Here's how the part is built. I have some questions about the finished solid (model axes, mm). Face numbers are marked on the shaded views. A direction names the side the tool comes from. Coordinates: 2 decimals unless noted, no trailing zeros. Order: outer loops, then holes, each group sorted by start corner. A loop starts at its lowest first (then second) coordinate and runs counter-clockwise, first axis right, second up. Notation, with made-up numbers: (-2, 45.25) - (16, 45.25) arc R24 ccw to (16, 76.25) - close; hole circle Ø1 at (23, -5.75). An arc over 180 degrees is marked (long way). Answer in a Markdown table with one row per item. Add a question column.
Item 1: If I drill on line 1 along X through (y, z) = (172, 53); line 2 along Z through (x, y) = (26.5, 202.5), over which ranges is the centre line in solid material (lowest first)? Write a range as from..to.
Item 2: I want a section at C-C (z = -3). Please give me the cut outline in (x, y), plus the area to 3 significant figures.
Item 3: Will these pins go through, and if not, where does the flat tip stop? pin 1 Ø12 at (x, z) = (34, -24.5) entering from +Y; pin 2 Ø2 at (x, y) = (55.5, 202.5) entering from +Z.
Item 4: I want a section at A-A (y = 42). Please give me the cut outline in (x, z), plus the area to 3 significant figures.
Item 5: I want a section at B-B (x = 53). Please give me the cut outline in (y, z).
Item 6: On a 3-axis mill with a long thin cutter (end or side, diameter ignored), from which of +Z, -Z, +X, -X, +Y, -Y can I reach the whole of each face in a straight line? I mean the marked faces 1 and 2. Say none if no direction works.
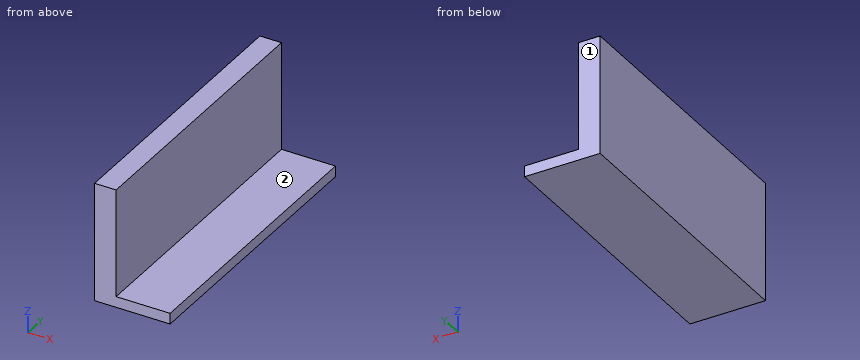
Autodesk Inventor part; units mm, degrees
ref_plane "YZ Plane" through (0, 0, 0) normal (1, 0, 0) x (0, 1, 0)
ref_plane "XZ Plane" through (0, 0, 0) normal (0, 1, 0) x (-1, 0, 0)
ref_plane "XY Plane" through (0, 0, 0) normal (0, 0, 1) x (1, 0, 0)
sketch "Sketch1" plane through (0, 0, 0) normal (0, 1, 0) x (-1, 0, 0)
  line L0 (-3.913, 66.9565) -> (-23.913, 66.9565)
  line L1 (-23.913, 66.9565) -> (-23.913, -43.0435)
  line L2 (-23.913, -43.0435) -> (-3.913, -43.0435)
  line L3 (-3.913, -43.0435) -> (-3.913, 66.9565)
  line L4 (53.6957, 6.9565) -> (-3.913, 6.9565)
  line L5 (-3.913, 6.9565) -> (-3.913, -18.0435)
  line L6 (-3.913, -18.0435) -> (48.6957, -18.0435)
  point P0 (0, 0)
  dimension "d0" = 110
  dimension "d1" = 20
  dimension "d3" = 60
extrude "Extrusion1" add sketch "Sketch1" along normal blind 260
chamfer "Chamfer1" [suppressed]
sketch "Sketch2" plane through (23.913, 0, 66.9565) normal (1, 0, 0) x (0, 0, -1)
  line L0 (110, 0) -> (110, 260)
  line L1 (110, 0) -> (0, 0)
  line L2 (110, 260) -> (100, 260)
  line L3 (100, 260) -> (100, 0)
  line L4 (100, 0) -> (110, 0)
  line L5 (110, 0) -> (110, 260)
  point P0 (100, 260)
  dimension "d9" = 10
extrude "Extrusion2" add sketch "Sketch2" along normal blind 50
sketch "Sketch4" plane through (3.913, 0, 66.9565) normal (0, 0, 1) x (1, 0, 0)
  circle A0 centre (60, 232) radius 84.5704
  point P0 (-3.913, 0)
extrude "Extrusion4" [suppressed]
sketch "Sketch5" plane through (3.913, 0, -15.0435) normal (0, 0, 1) x (1, 0, 0)
  arc A0 (0, 172.4) -> (15.6361, 160) centre (60, 232) ccw
  circle A1 centre (60, 232) radius 37.4531
  point P0 (-3.913, 0)
  point P1 (20, 162.1931)
extrude "Extrusion5" [suppressed]
properties part number "SecondSpindleOsnova" material "Aluminum 6061-AHC"
Values follow:
| question | item | result |
|---|---|---|
| 1 | line 1 | x = 3.91..23.91 |
| 1 | line 2 | z = -43.04..-33.04 |
| 2 | outline | (3.91, 0) - (23.91, 0) - (23.91, 260) - (3.91, 260) - close |
| 2 | area | 5,200 mm^2 |
| 3 | pin 1 | passes through |
| 3 | pin 2 | stops at z = -33.04 |
| 4 | outline | (3.91, -43.04) - (73.91, -43.04) - (73.91, -33.04) - (23.91, -33.04) - (23.91, 66.96) - (3.91, 66.96) - close |
| 4 | area | 2,700 mm^2 |
| 5 | outline | (0, -43.04) - (260, -43.04) - (260, -33.04) - (0, -33.04) - close |
| 6 | face 1 | +Z, -Z, +X, -X, +Y |
| 6 | face 2 | +Z, +X, +Y, -Y |
